Read the model definition and answer for the solid it produces. Units are mm, in the model's axes. A direction names the side the tool comes from. Coordinates: 2 decimals unless noted, no trailing zeros. Write each loop counter-clockwise with the first axis right and the second up, starting at its lowest first coordinate (ties: lowest second). Pieces come first, ordered by that corner, then holes. Notation, with made-up numbers: M 65,24.5 L 124,24.5 A17 cw 124,54.5 Z; hole C 41,-6.5 d3. An arc over 180 degrees is marked long. Write item = value, one per line.
from build123d import *

# Parameters (mm, degrees)
CUT_EXTRUDE1_DEPTH = 1
FILLET1_R          = 0.6


with BuildPart() as part:
    # Sketch1 → Revolve1 (revolve)
    with BuildSketch(Plane.XY, mode=Mode.PRIVATE) as revolve1_sk:
        Polygon((0, 0), (0, 10.12), (2.5, 10.12), (2.5, 8), (1.25, 8), (1.25, 0), align=None)
    revolve(revolve1_sk.sketch.rotate(Axis((0, 0, 0), (0, 1, 0)), 90), axis=Axis((0, 0, 0), (0, 1, 0)))

    # Sketch2 → Cut-Extrude1 (cut)
    with BuildSketch(Plane(origin=(0, 10.12, 0), x_dir=(1, 0, 0), z_dir=(0, 1, 0))):
        Polygon((-0.3, 0.3), (-1.35, 0.3), (-1.35, -0.3), (-0.3, -0.3), (-0.3, -1.35), (0.3, -1.35), (0.3, -0.3), (1.35, -0.3), (1.35, 0.3), (0.3, 0.3), (0.3, 1.35), (-0.3, 1.35), align=None)
    extrude(amount=-CUT_EXTRUDE1_DEPTH, mode=Mode.SUBTRACT)

    # Fillet1
    fillet1_edges = [part.edges().sort_by_distance(p)[0] for p in [
        (0, 10.12, 2.5),
    ]]
    fillet(fillet1_edges, radius=FILLET1_R)


solid = part.part
Item 1: Consider line 1 along Y through (x, z) = (0, -0.6); line 2 along X through (y, z) = (9.75, 0.45); line 3 along Y through (x, z) = (0, 1.9). Determine where each line is inside the solid, lowest interval first. Write a range as from..to.
Worked answers:
line_1 = 0..9.12
line_2 = -2.41..-0.3, 0.3..2.41
line_3 = 8..10.12
Item 2: Flat-ended cylindrical pins translate along their axes: pin 1 (0.8 mm diameter, centred on x = -0.5, y = 9.5, fed in from -Z); pin 2 (0.7 mm diameter, centred on y = 10, z = 0, fed in from -X); pin 3 (3 mm diameter, centred on y = 5, z = -1.5, fed in from -X). Find the tip coordinate at first contact, or state that the pin passes through.
Worked answers:
pin_1 = -2.5
pin_2 = -2.49
pin_3 = -1.25
Item 3: Find section A-A (x = 0). Determine the outline of the cut face in (y, z), and give its area (3 significant figures).
Worked answers:
outline = M 0,-1.25 L 8,-1.25 L 8,-2.5 L 9.52,-2.5 A0.6 ccw 10.12,-1.9 L 10.12,-1.35 L 9.12,-1.35 L 9.12,1.35 L 10.12,1.35 L 10.12,1.9 A0.6 ccw 9.52,2.5 L 8,2.5 L 8,1.25 L 0,1.25 Z
area = 27.7 mm²
Item 4: Which of the six approach directions +Z, -Z, +X, -X, +Y, -Y give full straight-line access (tool end or side, diameter ignored) to faces 4 (the face through (0.8, 9.6, -0.3)), 5 (the face through (-0.45, 10.12, -0.45))?
Worked answers:
face_4 = +Y
face_5 = +Z, -Z, +X, -X, +Y
Item 5: Find section C-C (y = 8.5). Determine the outline of the cut face in (x, z).
Worked answers:
outline = C 0,0 d5
Item 6: Find section D-D (y = 6.25). Determine the outline of the cut face in (x, z).
Worked answers:
outline = C 0,0 d2.5
Item 7: Find section B-B (z = 0). Determine the outline of the cut face in (x, y).
Worked answers:
outline = M -2.5,8 L -1.25,8 L -1.25,0 L 1.25,0 L 1.25,8 L 2.5,8 L 2.5,9.52 A0.6 ccw 1.9,10.12 L 1.35,10.12 L 1.35,9.12 L -1.35,9.12 L -1.35,10.12 L -1.9,10.12 A0.6 ccw -2.5,9.52 Z
Item 8: For a pull along X with two mould halves and no side action, classify faces 1 (the face through (-1, 8, -1)), 2 (the face through (-0.05, 3.94, 1.25)), 3 (the face through (0, 9.12, 0)) as released by +X, released by -X, zero draft, split by the parting line, or undercut.
Worked answers:
face_1 = zero draft
face_2 = split by the parting line
face_3 = undercut
